```python
from build123d import *

# Parameters (mm, degrees)
F1_DEPTH = 35
F2_W     = 24
F2_H     = 24
F3_DEPTH = 25.5
F5_D     = 6.5
F5_DEPTH = 35
F5_TIP   = 1.9527970118
F7_DEPTH = 8
F9_DEPTH = 8


with BuildPart() as f1:
    # F0 (on Top) → F1 (new body)
    with BuildSketch(Plane.XY):
        Polygon((-125, -17.5), (125, -17.5), (90, 17.5), (-125, 17.5), align=None)
    extrude(amount=F1_DEPTH)

    # F2 (on face) → F3 (cut)
    with BuildSketch(Plane(origin=(-125, 0, 0), x_dir=(0, -1, 0), z_dir=(-1, 0, 0))):
        with Locations((0, 17.5)):
            Rectangle(F2_W, F2_H)
    extrude(amount=-F3_DEPTH, mode=Mode.SUBTRACT)

    # F5
    with Locations(Plane.XY.offset(35)):
        with Locations((52.5, 0), (-70, 0)):
            Hole(F5_D / 2, depth=F5_DEPTH)
            with Locations((0, 0, -(F5_DEPTH + F5_TIP / 2))):  # 118° drill point
                Cone(0, F5_D / 2, F5_TIP, mode=Mode.SUBTRACT)

    # F6 (on face) → F7 (join)
    with BuildSketch(Plane(origin=(0, 0, 0), x_dir=(1, 0, 0), z_dir=(0, 0, -1))):
        with BuildLine():
            Line((98.6611652352, -8.8388347648), (116.3388347648, 8.8388347648))
            ThreePointArc((116.3388347648, 8.8388347648), (98.6611652352, 8.8388347648), (98.6611652352, -8.8388347648))
        make_face()
    extrude(amount=F7_DEPTH)

    # F8 (on face) → F9 (join)
    with BuildSketch(Plane(origin=(0, 0, 0), x_dir=(1, 0, 0), z_dir=(0, 0, -1))):
        with BuildLine():
            ThreePointArc((-125, -12.5), (-116.1611652352, -8.8388347648), (-112.5, 0))
            ThreePointArc((-112.5, 0), (-116.1611652352, 8.8388347648), (-125, 12.5))
            Line((-125, 12.5), (-125, -12.5))
        make_face()
    extrude(amount=F9_DEPTH)


solid = f1.part
```
Build history of the part. All positions in model axes, mm. A direction names the side the tool comes from. Coordinates: 2 decimals unless noted, no trailing zeros. Write each loop counter-clockwise with the first axis right and the second up, starting at its lowest first coordinate (ties: lowest second). Pieces come first, ordered by that corner, then holes.
1. Band-saw the part on B-B, the plane x = 52.5. Give the cut face in (y, z), and give its area (4 significant figures).
Answer block:
outline: (-17.5, 0) - (-3.25, 0) - (-3.25, 35) - (-17.5, 35) - close; (3.25, 0) - (17.5, 0) - (17.5, 35) - (3.25, 35) - close
area: 997.5 mm2
2. Drill centre lines: probe 1 along Y at (x, z) = (-70, 23.5); probe 2 along X at (y, z) = (0, 24); probe 3 along Z at (x, y) = (-11, 9). Where is each one in solid material? Low to high.
Answer block:
probe 1: y = -17.5 to -3.25, 3.25 to 17.5
probe 2: x = -99.5 to -73.25, -66.75 to 49.25, 55.75 to 107.5
probe 3: z = 0 to 35
3. Band-saw the part on A-A, the plane z = 15.5. Give the cut face in (x, y).
Answer block:
outline: (-125, -17.5) - (125, -17.5) - (90, 17.5) - (-125, 17.5) - (-125, 12) - (-99.5, 12) - (-99.5, -12) - (-125, -12) - close; hole circle Ø6.5 at (-70, 0); hole circle Ø6.5 at (52.5, 0)
4. Band-saw the part on C-C, the plane x = 107.5. Give the cut face in (y, z), and give its area (4 significant figures).
Answer block:
outline: (-17.5, 0) - (-12.5, 0) - (-12.5, -8) - (0, -8) - (0, 35) - (-17.5, 35) - close
area: 712.5 mm2
5. Pull direction Z, two halves, no side cores. Call faces 4 (the flat face through (-112, 12, 17)), 5 (the flat face through (107.7, -0.2, 13.2)), 6 (the flat face through (-112, -12, 17)), 7 (the flat face through (-2, 0, 0)): released by +Z, released by -Z, zero draft, split by the parting line, or undercut.
Answer block:
face 4: undercut
face 5: zero draft
face 6: undercut
face 7: released by -Z
6. Band-saw the part on D-D, the plane y = 6. Give the cut face in (x, z).
Answer block:
outline: (-125, -8) - (-114.03, -8) - (-114.03, 0) - (96.53, 0) - (96.53, -8) - (101.5, -8) - (101.5, 35) - (-125, 35) - (-125, 29.5) - (-99.5, 29.5) - (-99.5, 5.5) - (-125, 5.5) - close
7. Drop flat-ended pins along their axis: pin 1 (10.5 mm diameter, centred on x = -70, y = 0, fed in from -Z); pin 2 (6 mm diameter, centred on y = 5.5, z = 20, fed in from -X). Give the stop position or say it passes through.
Answer block:
pin 1: stops at z = 0
pin 2: stops at x = -99.5
8. 3-axis set-ups, long thin cutter, end or side, ignore diameter. For faces 1 (the cylindrical face through (98.858, -9.031, -3.944)), 2 (the flat face through (103, -4, -8)), 3 (the flat face through (-99.5, 0, 18)): which of +Z, -Z, +X, -X, +Y, -Y reach the whole face in a straight line?
Answer block:
face 1: -Z
face 2: -Z, +X, -X, +Y, -Y
face 3: -X
